Autodesk Inventor part; units mm, degrees
ref_plane "YZ Plane" through (0, 0, 0) normal (1, 0, 0) x (0, 1, 0)
ref_plane "XZ Plane" through (0, 0, 0) normal (0, 1, 0) x (-1, 0, 0)
ref_plane "XY Plane" through (0, 0, 0) normal (0, 0, 1) x (1, 0, 0)
sketch "Sketch1" plane through (0, 0, 0) normal (0, 0, 1) x (1, 0, 0)
  line L0 (-22.7093, 18.0885) -> (27.2907, 18.0885)
  line L1 (27.2907, 18.0885) -> (27.2907, -31.9115)
  line L2 (27.2907, -31.9115) -> (-22.7093, -31.9115)
  line L3 (-22.7093, -31.9115) -> (-22.7093, 18.0885)
  point P0 (0, 0)
  dimension "d0" = 50
  dimension "d1" = 50
extrude "Extrusion1" add sketch "Sketch1" along normal blind 10
sketch "Sketch3" plane through (0, 0, 10) normal (0, 0, 1) x (1, 0, 0)
  line L0 (-17.7093, 13.0885) -> (-9.0593, 13.0885)
  line L1 (-9.0593, 13.0885) -> (-9.0593, 4.4385)
  line L2 (-9.0593, 4.4385) -> (-17.7093, 4.4385)
  line L3 (-17.7093, 4.4385) -> (-17.7093, 13.0885)
  line L4 (-22.7093, 18.0885) -> (-22.7093, -31.9115)
  line L5 (27.2907, 18.0885) -> (-22.7093, 18.0885)
  line L6 (13.6407, 13.0885) -> (22.2907, 13.0885)
  line L7 (22.2907, 13.0885) -> (22.2907, 4.4385)
  line L8 (22.2907, 4.4385) -> (13.6407, 4.4385)
  line L9 (13.6407, 4.4385) -> (13.6407, 13.0885)
  line L10 (-17.7093, -18.2615) -> (-9.0593, -18.2615)
  line L11 (-9.0593, -18.2615) -> (-9.0593, -26.9115)
  line L12 (-9.0593, -26.9115) -> (-17.7093, -26.9115)
  line L13 (-17.7093, -26.9115) -> (-17.7093, -18.2615)
  line L14 (27.2907, -31.9115) -> (27.2907, 18.0885)
  line L15 (-22.7093, -31.9115) -> (27.2907, -31.9115)
  point P0 (0, 0)
  dimension "d8" = 5
  dimension "d9" = 5
  dimension "d10" = 8.65
  dimension "d11" = 8.65
  dimension "d12" = 5
  dimension "d13" = 8.65
  dimension "d14" = 8.65
  dimension "d15" = 5
  dimension "d16" = 5
  dimension "d17" = 5
  dimension "d18" = 8.65
  dimension "d19" = 8.65
extrude "Extrusion2" add sketch "Sketch3" along normal blind 15 contours L0 L1 L2 L3 | L6 L7 L8 L9 | L10 L11 L12 L13
equation "\"d13\" = d10"
equation "\"d15\" = d12"
equation "\"d16\" = d8"
equation "\"d19\" = d18"
properties part number "final_beam_cube_top"
Source: CAD feature listing. Evaluate the final solid. Frame: model axes, mm. A direction names the side the tool comes from. Give positions to 0.01 mm unless a question says otherwise; leave off trailing zeros. Loops run counter-clockwise (first coordinate to the right, second up) from the corner with the lowest first, then second, coordinate; pieces in that order, holes last. Notation, with made-up numbers: (33, 79) - (62, 79) arc R20 cw to (62, 93) - close; hole circle Ø11 at (12.5, 5.25). An arc over 180 degrees is marked (long way). Use CSV: the item, a comma, the result in double quotes. Start each with the question number.
1. Section B-B (x = -16). Output: boundary loops of the cut face in (y, z), then the cut area to 4 significant figures.
2. Draft query along X for faces 1 (the flat face through (27.291, -7, 5)), 2 (the flat face through (18, 4.438, 17)), 3 (the flat face through (-9.059, 9, 17)). Return one class per face: +X half, -X half, draft (parallel to the pull), parting line (faces both ways), or undercut.
3. Section C-C (y = 7). Output: boundary loops of the cut face in (x, z), then the cut area to 4 significant figures.
4. Section A-A (z = 14.75). Output: boundary loops of the cut face in (x, y), then the cut area to 3 significant figures.
5. Pin query (flat end, axial travel): pin 1 (2.5 mm diameter, centred on x = -13, z = 16.5, fed in from +Y); pin 2 (1 mm diameter, centred on x = 17, y = -4, fed in from -Z); pin 3 (4.5 mm diameter, centred on y = 11, z = 16, fed in from +X); pin 4 (2 mm diameter, centred on x = 8, y = -25, fed in from +Z). Return the tip coordinate at first contact, or that it passes through.
6. Ray query, L1, parallel to X at y = 10.5, z = 10.75; L2, parallel to Y at x = -9.5, z = 11; L3, parallel to Z at x = -6, y = 11. Return the intervals inside material, ascending.
7. Reachability of faces 4 (the flat face through (22.291, 9, 17)), 5 (the flat face through (-17.709, 9, 17)), 6 (the flat face through (-13, 13.088, 17)) from +Z, -Z, +X, -X, +Y, -Y: full face, straight path, thin tool, end or side. Return the list, or none.
8. Section D-D (y = -25). Output: boundary loops of the cut face in (x, z), then the cut area to 3 significant figures.
Response:
1,outline,"(-31.91, 0) - (18.09, 0) - (18.09, 10) - (13.09, 10) - (13.09, 25) - (4.44, 25) - (4.44, 10) - (-18.26, 10) - (-18.26, 25) - (-26.91, 25) - (-26.91, 10) - (-31.91, 10) - close"
1,area,"759.5 mm²"
2,face 1,"+X half"
2,face 2,"draft"
2,face 3,"undercut"
3,outline,"(-22.71, 0) - (27.29, 0) - (27.29, 10) - (22.29, 10) - (22.29, 25) - (13.64, 25) - (13.64, 10) - (-9.06, 10) - (-9.06, 25) - (-17.71, 25) - (-17.71, 10) - (-22.71, 10) - close"
3,area,"759.5 mm²"
4,outline,"(-17.71, -26.91) - (-9.06, -26.91) - (-9.06, -18.26) - (-17.71, -18.26) - close; (-17.71, 4.44) - (-9.06, 4.44) - (-9.06, 13.09) - (-17.71, 13.09) - close; (13.64, 4.44) - (22.29, 4.44) - (22.29, 13.09) - (13.64, 13.09) - close"
4,area,"224 mm²"
5,pin 1,"y = 13.09"
5,pin 2,"z = 0"
5,pin 3,"x = 22.29"
5,pin 4,"z = 10"
6,L1,"-17.71 to -9.06, 13.64 to 22.29"
6,L2,"-26.91 to -18.26, 4.44 to 13.09"
6,L3,"0 to 10"
7,face 4,"+Z, +X, +Y, -Y"
7,face 5,"+Z, -X, +Y, -Y"
7,face 6,"+Z, +X, -X, +Y"
8,outline,"(-22.71, 0) - (27.29, 0) - (27.29, 10) - (-9.06, 10) - (-9.06, 25) - (-17.71, 25) - (-17.71, 10) - (-22.71, 10) - close"
8,area,"630 mm²"
